```python
from build123d import *

# Parameters (mm, degrees)
SKETCH1_W           = 45
SKETCH1_H           = 45
BOSS_EXTRUDE1_DEPTH = 2
SKETCH2_W           = 7
SKETCH2_H           = 2.72647494
SKETCH2_H_2         = 3
SKETCH2_W_2         = 3
SKETCH2_H_3         = 7
CUT_EXTRUDE1_DEPTH  = 10


with BuildPart() as part:
    # Sketch1 → Boss-Extrude1 (new body)
    with BuildSketch(Plane.XY):
        Rectangle(SKETCH1_W, SKETCH1_H)
    extrude(amount=BOSS_EXTRUDE1_DEPTH)

    # Sketch2 → Cut-Extrude1 (cut)
    with BuildSketch(Plane.XY.offset(2)):
        Polygon((-22.5, -12.5), (-22.5, -22.5), (-19.5, -22.5), (-19.5, -19.77352506), (-19.5, -12.5), align=None)
        with Locations((-16, -21.13676253)):
            Rectangle(SKETCH2_W, SKETCH2_H)
        Polygon((19.5, -22.5), (22.5, -22.5), (22.5, -12.5), (19.5, -12.5), (19.5, -19.5), align=None)
        with Locations((16, -21)):
            Rectangle(SKETCH2_W, SKETCH2_H_2)
        Polygon((-12.5, 22.5), (-22.5, 22.5), (-22.5, 19.5), (-19.5, 19.5), (-12.5, 19.5), align=None)
        with Locations((-21, 16)):
            Rectangle(SKETCH2_W_2, SKETCH2_H_3)
        Polygon((22.5, 12.5), (22.5, 22.5), (19.5, 22.5), (19.5, 19.5), (19.5, 12.5), align=None)
        with Locations((16, 21)):
            Rectangle(SKETCH2_W, SKETCH2_H_2)
    extrude(amount=-CUT_EXTRUDE1_DEPTH, mode=Mode.SUBTRACT)


solid = part.part
```
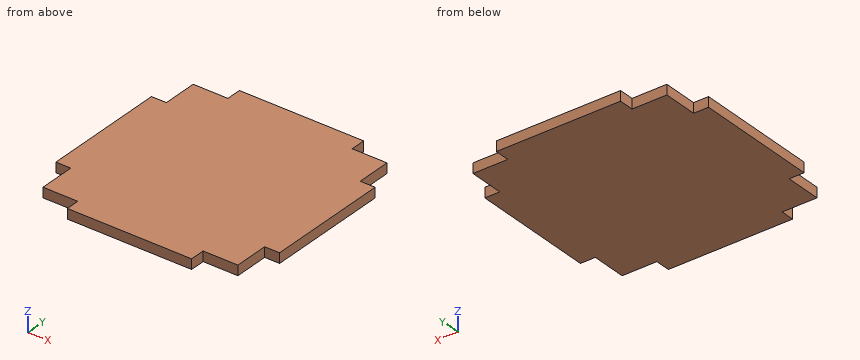
Source: CAD feature listing. Evaluate the final solid. Frame: model axes, mm. Round coordinates to 2 decimals unless told otherwise and drop trailing zeros. Order: outer loops, then holes, each group sorted by start corner. A loop starts at its lowest first (then second) coordinate and runs counter-clockwise, first axis right, second up. Notation, with made-up numbers: (59.5, 75.5) -> (90.5, 75.5) arc R8 cw to (90.5, 79.5) -> close; hole circle Ø3 at (17, 89.25). An arc over 180 degrees is marked (long way). One line per item, written item: value. Start each with the question number.
Q1. Material intervals for probe 1 along X at (y, z) = (-16.5, 0.2); probe 2 along Y at (x, z) = (-16.5, 1.25), sorted ascending.
Q2. Section query B-B (x = -16). Return the cut outline in (y, z), plus the area to 3 significant figures.
Q3. Section query C-C (y = -17.5). Return the cut outline in (x, z).
Q4. Pin query (flat end, axial travel): pin 1 (1 mm diameter, centred on x = -21.5, z = 1, fed in from -Y); pin 2 (1 mm diameter, centred on x = -20.5, z = 0.5, fed in from +Y); pin 3 (1 mm diameter, centred on y = 21, z = 1, fed in from -X). Return the tip coordinate at first contact, or that it passes through.
Q5. Section query A-A (z = 0.4). Return the cut outline in (x, y).
Findings below:
1. probe 1: -19.5 to 19.5
1. probe 2: -19.77 to 19.5
2. outline: (-19.77, 0) -> (19.5, 0) -> (19.5, 2) -> (-19.77, 2) -> close
2. area: 78.5 mm²
3. outline: (-19.5, 0) -> (19.5, 0) -> (19.5, 2) -> (-19.5, 2) -> close
4. pin 1: y = -12.5
4. pin 2: y = 12.5
4. pin 3: x = -12.5
5. outline: (-22.5, -12.5) -> (-19.5, -12.5) -> (-19.5, -19.77) -> (-12.5, -19.77) -> (-12.5, -22.5) -> (12.5, -22.5) -> (12.5, -19.5) -> (19.5, -19.5) -> (19.5, -12.5) -> (22.5, -12.5) -> (22.5, 12.5) -> (19.5, 12.5) -> (19.5, 19.5) -> (12.5, 19.5) -> (12.5, 22.5) -> (-12.5, 22.5) -> (-12.5, 19.5) -> (-19.5, 19.5) -> (-19.5, 12.5) -> (-22.5, 12.5) -> close
